Study the drawing (mm; zero at the part's minimum x, y, z) and answer. A direction names the side the tool comes from. Round coordinates to 2 decimals unless told otherwise and drop trailing zeros. Write each loop counter-clockwise with the first axis right and the second up, starting at its lowest first coordinate (ties: lowest second). Pieces come first, ordered by that corner, then holes. Notation, with made-up numbers: M 52.5,45 L 75.5,45 A14 ccw 75.5,65 Z; hole C -6,62 d9. An arc over 180 degrees is marked long. Write each question's results on one line, items separated by ' | '.
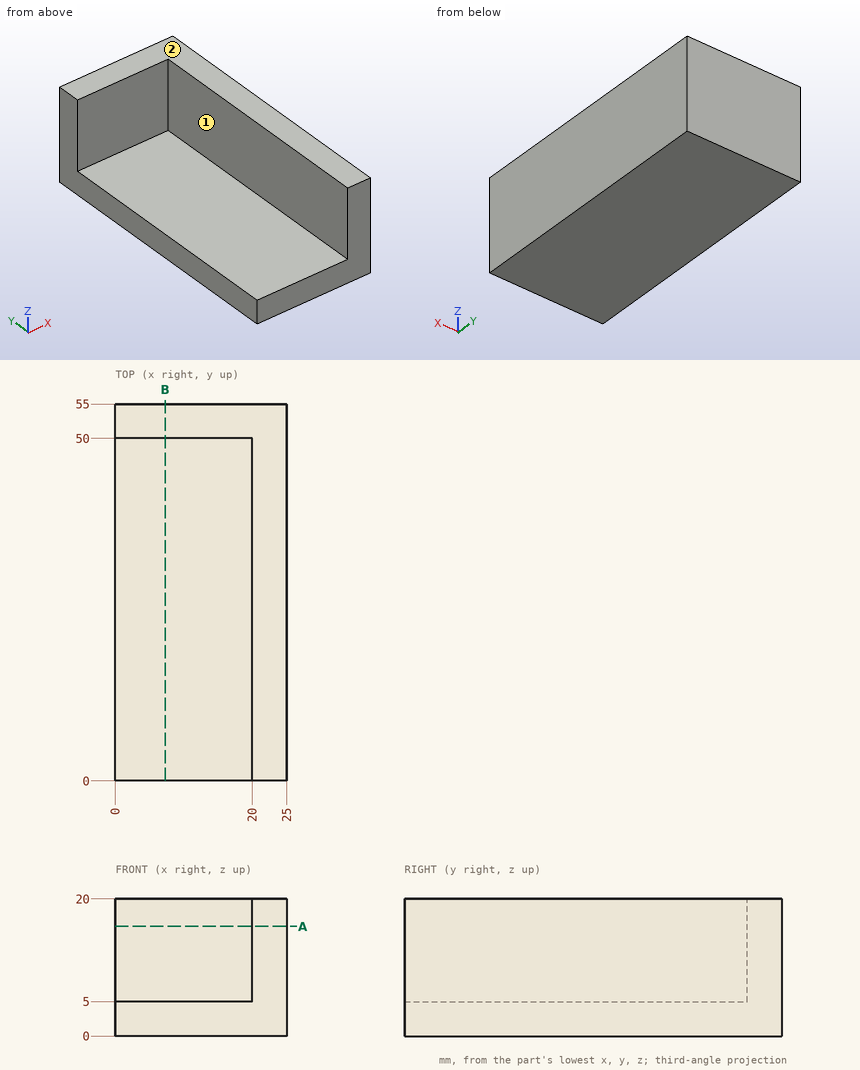
1) Section B-B (x = 7.25) is taken. Determine the outline of the cut face in (y, z), then the cut area to 3 significant figures.
Return value:
outline: M 0,0 L 55,0 L 55,20 L 50,20 L 50,5 L 0,5 Z | area: 350 mm²
2) Section A-A (z = 16) is taken. Determine the outline of the cut face in (x, y), then the cut area to 3 significant figures.
Return value:
outline: M 0,50 L 20,50 L 20,0 L 25,0 L 25,55 L 0,55 Z | area: 375 mm²
3) Find the intervals of material crossed by line 1 (X direction, y = 46, z = 10.5); line 2 (Y direction, x = 14.5, z = 11.5); line 3 (Z direction, x = 17, y = 45.5), in increasing order.
Return value:
line 1: 20 to 25 | line 2: 50 to 55 | line 3: 0 to 5
4) A tool of negligible diameter and unlimited length cuts with its end or side. For the marked faces 1 and 2, from which of +Z, -Z, +X, -X, +Y, -Y can it reach the whole face along a straight path? Write none if from no direction.
Return value:
face 1: +Z, -X, -Y | face 2: +Z, +X, -X, +Y, -Y
5) Each of these flat-tipped pins is pushed along its axis until it touches: pin 1 (1.5 mm diameter, centred on x = 9.5, y = 47, fed in from +Z); pin 2 (8 mm diameter, centred on x = 11.5, y = 39, fed in from -Z); pin 3 (2 mm diameter, centred on x = 11, z = 13, fed in from -Y); pin 4 (4.5 mm diameter, centred on y = 28.5, z = 16, fed in from -X). Where does it stop, or does it pass through?
Return value:
pin 1: z = 5 | pin 2: z = 0 | pin 3: y = 50 | pin 4: x = 20
